Check sheet for the modelled part. Datum: model origin and axes. Units: mm. Face numbers are marked on the shaded views. Give positions to 0.01 mm unless a question says otherwise; leave off trailing zeros. Write each loop counter-clockwise with the first axis right and the second up, starting at its lowest first coordinate (ties: lowest second). Pieces come first, ordered by that corner, then holes. Notation, with made-up numbers: M 65.25,15 L 69.25,15 A30 cw 69.25,41 Z; hole C 69.5,33 d7. An arc over 180 degrees is marked long. Write item = value, one per line. Start each with the question number.
1) Cross-section at A-A, the plane x = 0. Record the cut outline in (y, z).
2) Scan lines: line 1 along Y through (x, z) = (0.25, 16.75); line 2 along Z through (x, y) = (1.25, -4.5); line 3 along Y through (x, z) = (8.75, 20.75). Record each from-to range of solid material in increasing order. Write a range as [from, to].
3) Go/stop test with flat-tipped pins: pin 1 (5.5 mm diameter, centred on x = -1, y = -2.5, fed in from +Z); pin 2 (4 mm diameter, centred on x = -3, z = 14.5, fed in from -Y); pin 3 (5 mm diameter, centred on y = 6.5, z = 26, fed in from -X). Record where each tip stops, or that it passes through.
4) Cross-section at C-C, the plane z = 3.75. Record the cut outline in (x, y), plus the area to 3 significant figures.
5) Mould release check, pull along X, two halves, no side actions. Record for the marked faces 1, 2 and 3: released by +X, released by -X, zero draft, split by the parting line, or undercut.
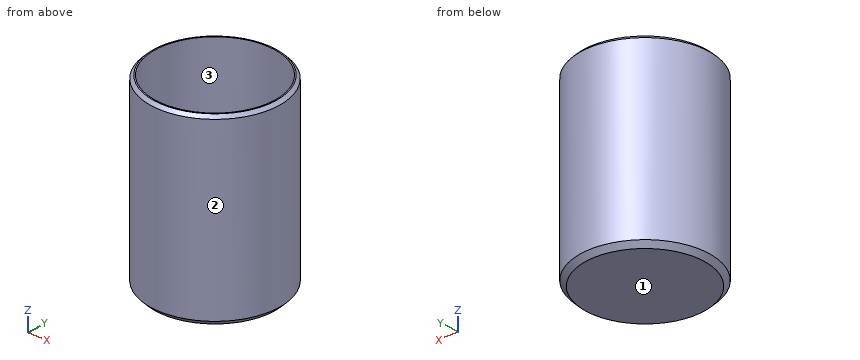
```python
from build123d import *

# Parameters (mm, degrees)
F0_R     = 9.75
F1_DEPTH = 0.5
F0_R_2   = 10.45
F2_DEPTH = 29.5
F3_SIZE  = 0.5
F4_SIZE  = 0.4
F5_SIZE  = 0.8


with BuildPart() as f1:
    # F0 (on Top) → F1 (new body)
    with BuildSketch(Plane.XY):
        Circle(F0_R)
    extrude(amount=F1_DEPTH)

    # F0 (on Top) → F2 (join)
    with BuildSketch(Plane.XY):
        Circle(F0_R_2)
        Circle(F0_R, mode=Mode.SUBTRACT)
    extrude(amount=F2_DEPTH)

    # F3
    f3_edges = [f1.edges().sort_by_distance(p)[0] for p in [
        (-10.45, 0, 29.5),
    ]]
    chamfer(f3_edges, length=F3_SIZE)

    # F4
    f4_edges = [f1.edges().sort_by_distance(p)[0] for p in [
        (-9.75, 0, 0.5),
    ]]
    chamfer(f4_edges, length=F4_SIZE)

    # F5
    f5_edges = [f1.edges().sort_by_distance(p)[0] for p in [
        (-10.45, 0, 0),
    ]]
    chamfer(f5_edges, length=F5_SIZE)


solid = f1.part
```
Reply:
q1.outline = M -10.45,0.8 L -9.65,0 L 9.65,0 L 10.45,0.8 L 10.45,29 L 9.95,29.5 L 9.75,29.5 L 9.75,0.9 L 9.35,0.5 L -9.35,0.5 L -9.75,0.9 L -9.75,29.5 L -9.95,29.5 L -10.45,29 Z
q2.line_1 = [-10.45, -9.75], [9.75, 10.45]
q2.line_2 = [0, 0.5]
q2.line_3 = [-5.71, -4.3], [4.3, 5.71]
q3.pin_1 = 0.5
q3.pin_2 = -10.4
q3.pin_3 = -9.65
q4.outline = C 0,0 d20.9; hole C 0,0 d19.5
q4.area = 44.4 mm2
q5.face_1 = zero draft
q5.face_2 = split by the parting line
q5.face_3 = undercut
